Build history of the part. All positions in model axes, mm. A direction names the side the tool comes from. Round coordinates to 2 decimals unless told otherwise and drop trailing zeros. Write each loop counter-clockwise with the first axis right and the second up, starting at its lowest first coordinate (ties: lowest second). Pieces come first, ordered by that corner, then holes.
from build123d import *

# Parameters (mm, degrees)
ESBO_O1_W                = 3.5
ESBO_O1_H                = 10
RESSALTO_EXTRUS_O1_DEPTH = 6
FILETE1_R                = 1.75


with BuildPart() as part:
    # Esboço1 → Ressalto-extrusão1 (new body)
    with BuildSketch(Plane.XY):
        Polygon((5.5, 32.5), (0, 32.5), (-5.5, 32.5), (-5.5, 26.5), (-13, 26.5), (-13, -32.5), (13, -32.5), (13, 26.5), (5.5, 26.5), align=None)
        with Locations((0, 15.5)):
            Rectangle(ESBO_O1_W, ESBO_O1_H, mode=Mode.SUBTRACT)
        with Locations((0, 0.5)):
            Rectangle(ESBO_O1_W, ESBO_O1_H, mode=Mode.SUBTRACT)
    extrude(amount=RESSALTO_EXTRUS_O1_DEPTH)

    # Filete1
    filete1_edges = [part.edges().sort_by_distance(p)[0] for p in [
        (-1.75, -4.5, 3),
        (1.75, -4.5, 3),
        (1.75, 5.5, 3),
        (-1.75, 5.5, 3),
        (1.75, 10.5, 3),
        (-1.75, 10.5, 3),
        (1.75, 20.5, 3),
        (-1.75, 20.5, 3),
    ]]
    fillet(filete1_edges, radius=FILETE1_R - 0.0001)  # a hair under: the kernel refuses the full size


solid = part.part
1) Pin check, flat tips, straight feed: pin 1 Ø1.8 at (x, z) = (8.5, 2) entering from +Y; pin 2 Ø1.8 at (y, z) = (29.5, 4.5) entering from -X. Stop position of each tip, or through.
Results:
pin 1: stops at y = 26.5
pin 2: stops at x = -5.5
2) Which spindle directions (+Z, -Z, +X, -X, +Y, -Y) get a long thin tool onto all of the face, cutting with end or side? Do faces 1 (the flat face through (0, 32.5, 3)), 2 (the flat face through (-9, 26.5, 3)), 3 (the flat face through (5.5, 29, 3)), 4 (the cylindrical face through (1.251, 4.974, 3.042)). Say none if no direction does.
Results:
face 1: +Z, -Z, +X, -X, +Y
face 2: +Z, -Z, -X, +Y
face 3: +Z, -Z, +X, +Y
face 4: +Z, -Z
3) Slice it at A-A (z = 3.9). Count the separate pieces of the cut face and the enclosed holes in it, plus the area to 3 significant figures.
Results:
separate pieces: 1
enclosed holes: 2
area: 1,540 mm2
4) Wall check: L1, parallel to X at y = 18.5, z = 1.4; L2, parallel to Y at x = -0.25, z = 0.6; L3, parallel to Y at x = -1, z = 3.4. Give the ranges that are in metal, low to high.
Results:
L1: x = -13 to -1.75, 1.75 to 13
L2: y = -32.5 to -4.48, 5.48 to 10.52, 20.48 to 32.5
L3: y = -32.5 to -4.19, 5.19 to 10.81, 20.19 to 32.5
5) Mould opens along X. For faces 5 (the flat face through (-5.5, 30, 3)), 6 (the cylindrical face through (-1.224, 5.001, 3.042)), 7 (the flat face through (9, 26.5, 3)) say: released by +X, released by -X, zero draft, split by the parting line, or undercut.
Results:
face 5: released by -X
face 6: undercut
face 7: zero draft
6) Slice it at B-B (x = 8.25). Write the cut outline in (y, z).
Results:
outline: (-32.5, 0) - (26.5, 0) - (26.5, 6) - (-32.5, 6) - close
